The listing builds one solid part. Answer for the finished solid, in the listing's coordinates (mm). A direction names the side the tool comes from. Coordinates: 2 decimals unless noted, no trailing zeros. Order: outer loops, then holes, each group sorted by start corner. A loop starts at its lowest first (then second) coordinate and runs counter-clockwise, first axis right, second up.
from build123d import *

# Parameters (mm, degrees)
SKETCH1_R                = 20
SKETCH1_R_2              = 25
BOSS_EXTRUDE1_DEPTH      = 4
BOSS_EXTRUDE2_DEPTH      = 19.1
SKETCH5_R                = 5.02
CUT_EXTRUDE1_DEPTH       = 49.2
SKETCH7_R                = 5
BOSS_EXTRUDE4_DEPTH      = 40.2
BOSS_EXTRUDE4_DEPTH_BACK = 2.2


with BuildPart() as part:
    # Sketch1 → Boss-Extrude1 (new body)
    with BuildSketch(Plane.XY):
        with Locations((-13.047428352, 181.745231989)):
            Circle(SKETCH1_R)
        with BuildLine():
            ThreePointArc((-15.752419285, 19.412915461), (0, 25), (15.752419285, 19.412915461))
            add(Edge.make_bspline(
                [(15.752419285, 19.412915461), (37.630116676, 100.741066361), (3.061753137, 169.892204032)],
                knots=[0, 0, 0, 1, 1, 1], degree=2))
            ThreePointArc((3.061753137, 169.892204032), (-10.099117092, 161.963739105), (-25, 165.709770319))
            add(Edge.make_bspline(
                [(-15.752419285, 19.412915461), (10.03237034, 99.240514814), (-25, 165.709770319)],
                knots=[0, 0, 0, 1, 1, 1], degree=2))
        make_face()
        Circle(SKETCH1_R_2)
    extrude(amount=BOSS_EXTRUDE1_DEPTH)

    # Sketch4 → Boss-Extrude2 (add)
    with BuildSketch(Plane.XY.offset(4)):
        with BuildLine():
            ThreePointArc((-15.752419292, 19.412915437), (1e-08, -24.999999987), (15.752419285, 19.412915461))
            add(Edge.make_bspline(
                [(15.752419285, 19.412915461), (32.045521078, 79.98089104), (17.031874688, 133.795114798)],
                knots=[0, 0, 0, 1, 1, 1], degree=2))
            add(Edge.make_bspline(
                [(-10.953146695, 130.455943826), (5.564580589, 116.540527234), (17.031874688, 133.795114798)],
                knots=[0, 0, 0, 1, 1, 1], degree=2))
            add(Edge.make_bspline(
                [(-10.953146695, 130.455943826), (3.367631556, 78.60702873), (-15.752419292, 19.412915437)],
                knots=[0, 0, 0, 1, 1, 1], degree=2))
        make_face()
    extrude(amount=BOSS_EXTRUDE2_DEPTH)

    # Mirror18: part across plane


with BuildPart() as part_1:
    add(part.part)
    add(part.part.mirror(Plane(origin=(4.301972293, 124.333028273, 23.1), x_dir=(1, 0, 0), z_dir=(0, 0, -1))))

    # Sketch5 → Cut-Extrude1 (cut)
    with BuildSketch(Plane.XY.offset(46.2)):
        Circle(SKETCH5_R)
    extrude(amount=-CUT_EXTRUDE1_DEPTH, mode=Mode.SUBTRACT)

    # Sketch7 → Boss-Extrude4 (add, two sides)
    with BuildSketch(Plane.XY.offset(4)) as boss_extrude4_sk:
        with Locations((-13.104058639, 181.741755044)):
            Circle(SKETCH7_R)
    extrude(amount=BOSS_EXTRUDE4_DEPTH)
    extrude(boss_extrude4_sk.sketch, amount=-BOSS_EXTRUDE4_DEPTH_BACK)


solid = part_1.part
1) Determine the mould class of faces 1 (the face through (-1.1, -4.9, 23.4)), 2 (the face through (2, 90, 0)) for opening direction Y: released by +Y, released by -Y, zero draft, split by the parting line, or undercut.
2) A tool of negligible diameter and unlimited length cuts with its end or side. For faces 3 (the face through (-13.75, 186.7, 22.83)), 4 (the face through (2, 90, 46.2)), from which of +Z, -Z, +X, -X, +Y, -Y can it reach the whole face along a straight path? Write none if from no direction.
3) Section B-B (z = 12) is taken. Give the number of separate pieces and of enclosed holes in the cut face, then the cut area to 3 significant figures.
4) Each of these flat-tipped pins is pushed along its axis until it touches: P1, Ø6, axis at y = 131, z = 26, coming from the +X side; P2, Ø1.5, axis at y = 66.5, z = 29, coming from the +X side; P3, Ø1.5, axis at x = 11.5, z = 14.5, coming from the +Y side. Where does it stop, or does it pass through?
5) Consider L1, parallel to Y at x = 2, z = 11; L2, parallel to X at y = 77, z = 37; L3, parallel to Y at x = -21, z = 44. Determine where each line is inside the solid, lowest interval first.
6) Section A-A (y = 0) is taken. Give the vertices of the cut face in (x, z), then the cut area to 3 significant figures.
Filled sheet:
1. face 1: undercut
1. face 2: zero draft
2. face 3: none
2. face 4: +Z, +X, -X, +Y, -Y
3. separate pieces: 2
3. enclosed holes: 1
3. area: 5,020 mm2
4. P1: stops at x = 18.55
4. P2: stops at x = 23.81
4. P3: stops at y = 128.15
5. L1: y = -24.92 to -4.6, 4.6 to 124.27
5. L2: x = -4.98 to 24.2
5. L3: y = -13.56 to 13.56, 157.65 to 200.1
6. outline: (-25, 0) - (-5.02, 0) - (-5.02, 46.2) - (-25, 46.2) - close; (5.02, 0) - (25, 0) - (25, 46.2) - (5.02, 46.2) - close
6. area: 1,850 mm2
